Source: CAD feature listing. Evaluate the final solid. Frame: model axes, mm. A direction names the side the tool comes from. Coordinates: 2 decimals unless noted, no trailing zeros. Write each loop counter-clockwise with the first axis right and the second up, starting at its lowest first coordinate (ties: lowest second). Pieces come first, ordered by that corner, then holes. Notation, with made-up numbers: (54, -34) - (66, -34) arc R29 ccw to (66, -10) - close; hole circle Ø11 at (19.5, -23). An arc over 180 degrees is marked (long way). One line per question, with ' | ' between items.
from build123d import *

# Parameters (mm, degrees)
SKETCH1_R            = 1.5
EXTRUDE1_DEPTH       = 8
CUT_SWEEP1_PITCH     = 0.5
SKETCH6_R            = 2.75
EXTRUDE2_DEPTH       = 3
CUT_EXTRUDE1_DEPTH   = 1.875
CHAMFER1_SIZE        = 0.275
SKETCH10_R           = 1.5
PARTIAL_THREAD_DEPTH = 8
CHAMFER2_SIZE        = 0.06


with BuildPart() as part:
    # Sketch1 → Extrude1 (new body)
    with BuildSketch(Plane.XY):
        Circle(SKETCH1_R)
    extrude(amount=-EXTRUDE1_DEPTH)

    # Cut-Sweep1: the profile of Sketch3 profile screwed along a right-hand helix of 17 turns, 6 arcs to a turn; built about Z, then put on its axis
    cut_sweep1_z = Axis((0, 0, 0), (0, 0, 1))
    cut_sweep1_corners = [(1.5003, 0, -0.437673205), (1.175240474, 0, -0.25), (1.175240474, 0, -0.1875), (1.5003, 0, 0.000173205)]
    with BuildLine(mode=Mode.PRIVATE) as cut_sweep1_profile:
        Line(cut_sweep1_corners[0], cut_sweep1_corners[1])
        Line(cut_sweep1_corners[1], cut_sweep1_corners[2])
        Line(cut_sweep1_corners[2], cut_sweep1_corners[3])
        Line(cut_sweep1_corners[3], cut_sweep1_corners[0])
    cut_sweep1_cap = Face(cut_sweep1_profile.wire())
    cut_sweep1_turn_angles = [0, 30, 60, 90, 120, 150, 180, 210, 240, 270, 300, 330, 360]
    cut_sweep1_turn_weights = [1, 0.8660254037844387, 1, 0.8660254037844387, 1, 0.8660254037844387, 1, 0.8660254037844387, 1, 0.8660254037844387, 1, 0.8660254037844387, 1]
    cut_sweep1_turn_rails = [Edge.make_bspline([Vector(p[0], p[1], 0).rotate(cut_sweep1_z, cut_sweep1_turn_angles[k]) / cut_sweep1_turn_weights[k] + Vector(0, 0, p[2] + CUT_SWEEP1_PITCH * cut_sweep1_turn_angles[k] / 360) for k in range(13)], [0, 0, 0, 1, 1, 2, 2, 3, 3, 4, 4, 5, 5, 6, 6, 6], 2, cut_sweep1_turn_weights) for p in cut_sweep1_corners]
    cut_sweep1_turn_sides = [Face.make_surface_from_curves(cut_sweep1_turn_rails[p[0]], cut_sweep1_turn_rails[p[1]]) for p in [(0, 1), (1, 2), (2, 3), (3, 0)]]
    cut_sweep1 = Plane(origin=(0, 0, 0), x_dir=(0, 1, 0), z_dir=(0, 0, -1)) * Solid(Shell([*[p.moved(Location((0, 0, CUT_SWEEP1_PITCH * i))) for i in range(17) for p in cut_sweep1_turn_sides], cut_sweep1_cap, cut_sweep1_cap.rotate(cut_sweep1_z, 6120).moved(Location((0, 0, CUT_SWEEP1_PITCH * 6120 / 360)))]))
    add(cut_sweep1, mode=Mode.SUBTRACT)

    # Sketch4 → Cut-Revolve1 (revolve, cut)
    with BuildSketch(Plane(origin=(0, 0, 0), x_dir=(0, 0, -1), z_dir=(1, 0, 0)), mode=Mode.PRIVATE) as cut_revolve1_sk:
        Polygon((0.405251783, 1.5), (0, 0.921240474), (0, 1.5), align=None)
    revolve(cut_revolve1_sk.sketch.rotate(Axis((0, 0, 0), (0, 0, -1)), 270), axis=Axis((0, 0, 0), (0, 0, -1)), mode=Mode.SUBTRACT)

    # Sketch6 → Extrude2 (add)
    with BuildSketch(Plane(origin=(0, 0, -8), x_dir=(-1, 0, 0), z_dir=(0, 0, -1))):
        Circle(SKETCH6_R)
    extrude(amount=EXTRUDE2_DEPTH)

    # Sketch7 → Cut-Extrude1 (cut)
    with BuildSketch(Plane(origin=(0, 0, -11), x_dir=(-1, 0, 0), z_dir=(0, 0, -1))):
        Polygon((0, 1.443375673), (-1.25, 0.721687836), (-1.25, -0.721687836), (0, -1.443375673), (1.25, -0.721687836), (1.25, 0.721687836), align=None)
    extrude(amount=-CUT_EXTRUDE1_DEPTH, mode=Mode.SUBTRACT)

    # Cut-Extrude2 cone 1 section (through the dimple's axis) → Cut-Extrude2 (revolve, cut)
    with BuildSketch(Plane(origin=(0, 0, -11), x_dir=(0, 1, 0), z_dir=(1, 0, 0))):
        Polygon((0, 0), (1.443375673, 0), (0, 1.443375673), align=None)
    revolve(axis=Axis((0, 0, -11), (0, 0, 1)), mode=Mode.SUBTRACT)

    # Chamfer1
    chamfer1_edges = [part.edges().sort_by_distance(p)[0] for p in [
        (2.75, 0, -8),
        (2.75, 0, -11),
    ]]
    chamfer(chamfer1_edges, length=CHAMFER1_SIZE)


with BuildPart() as body_2:
    # Sketch10 → partial thread (new body)
    with BuildSketch(Plane.XY.offset(-8)):
        Circle(SKETCH10_R)
    extrude(amount=PARTIAL_THREAD_DEPTH)

    # Chamfer2
    chamfer2_edges = [body_2.edges().sort_by_distance(p)[0] for p in [
        (-1.5, 0, 0),
    ]]
    chamfer(chamfer2_edges, length=CHAMFER2_SIZE)


with BuildPart() as part_1:
    add(part.part)

    # Combine1: union body 2
    add(body_2.part)


solid = part_1.part
Item 1: Pin query (flat end, axial travel): pin 1 Ø0.8 at (x, y) = (-0.5, 0.5) entering from -Z (3 decimals); pin 2 Ø2 at (x, z) = (-0.5, -3.5) entering from -Y; pin 3 Ø1.5 at (y, z) = (-1.5, -2) entering from +X. Return the tip coordinate at first contact, or that it passes through.
Check sheet entries:
pin 1: z = -9.125 | pin 2: y = -1.5 | pin 3: x = 1.3
Item 2: Access query for faces 5 (the face through (-0.63, 1.08, -10.08)), 6 (the face through (-2, 0, -8)). Directions: +Z, -Z, +X, -X, +Y, -Y. A direction counts if a zero-diameter tool reaches every point of the face in a straight line with its end or side. Return the directions, or none.
Check sheet entries:
face 5: -Z | face 6: +Z
Item 3: Cut plane A-A on y = 0. Return loops of the section in (x, z) (3 decimals).
Check sheet entries:
outline: (-2.75, -10.725) - (-2.475, -11) - (-1.443, -11) - (-1.25, -10.807) - (-1.25, -9.125) - (1.25, -9.125) - (1.25, -10.807) - (1.443, -11) - (2.475, -11) - (2.75, -10.725) - (2.75, -8.275) - (2.475, -8) - (1.5, -8) - (1.5, -0.06) - (1.44, 0) - (-1.44, 0) - (-1.5, -0.06) - (-1.5, -8) - (-2.475, -8) - (-2.75, -8.275) - close
Item 4: Ray query, line 1 along Z through (x, y) = (-1.8, -0.9); line 2 along X through (y, z) = (0.1, -10.5); line 3 along Z through (x, y) = (0.55, 0.5) (3 decimals). Return the intervals inside material, ascending. Write a range as [from, to].
Check sheet entries:
line 1: [-11, -8] | line 2: [-2.75, -1.25], [1.25, 2.75] | line 3: [-9.125, 0]
Item 5: Cut plane B-B on z = -7.5. Return loops of the section in (x, y), and give its area (3 significant figures).
Check sheet entries:
outline: circle Ø3 at (0, 0) | area: 7.07 mm²
Item 6: Mould query, pull axis X, two halves, no side actions, for faces 1 (the face through (0.63, -1.08, -10.08)), 2 (the face through (0.596, -2.685, -9.483)), 3 (the face through (-2, 0, -11)), 4 (the face through (0.616, 1.088, -10.076)). Classes: pulls with the +X half, pulls with the -X half, needs draft (parallel to the pull), parting line crosses it, or undercut.
Check sheet entries:
face 1: undercut | face 2: parting line crosses it | face 3: needs draft | face 4: undercut
